Here's the drawing with two shaded views (mm, measured from the low corner). I have some questions. Give positions to 0.01 mm unless a question says otherwise; leave off trailing zeros. Loops run counter-clockwise (first coordinate to the right, second up) from the corner with the lowest first, then second, coordinate; pieces in that order, holes last. Notation, with made-up numbers: (-26.75, 48.5) - (-5.75, 48.5) arc R9 cw to (-5.75, 54.5) - close; hole circle Ø11 at (-27.5, 72.25). An arc over 180 degrees is marked (long way). Write each question's results on one line, items separated by ' | '. Start each with the question number.
1) I want a section at B-B, the plane y = 19. Write out the boundary of the cut face in (x, z).
2) I want a section at C-C, the plane z = 0.6. Write out the boundary of the cut face in (x, y), and give its area (3 significant figures).
3) I'm going to push flat-ended pins straight in: pin 1 (0.7 mm diameter, centred on x = 1.5, z = 2, fed in from +Y); pin 2 (0.9 mm diameter, centred on y = 3.5, z = 2, fed in from -X); pin 3 (0.9 mm diameter, centred on y = 4, z = 2, fed in from +X); pin 4 (1.4 mm diameter, centred on x = 39, y = 22.5, fed in from +Z). Where does each tip first touch, or does it pass through?
4) I want a section at D-D, the plane y = 42. Write out the boundary of the cut face in (x, z), and give its area (3 significant figures).
5) I want a section at A-A, the plane x = 12.5. Write out the boundary of the cut face in (y, z), and give its area (3 significant figures).
6) If I drill on probe 1 along Y at (x, z) = (21, 0.9); probe 2 along X at (y, z) = (35.5, 1.6); probe 3 along Y at (x, z) = (25, 0.2), over which ranges is the centre line in solid material (lowest first)? Write a range as [from, to].
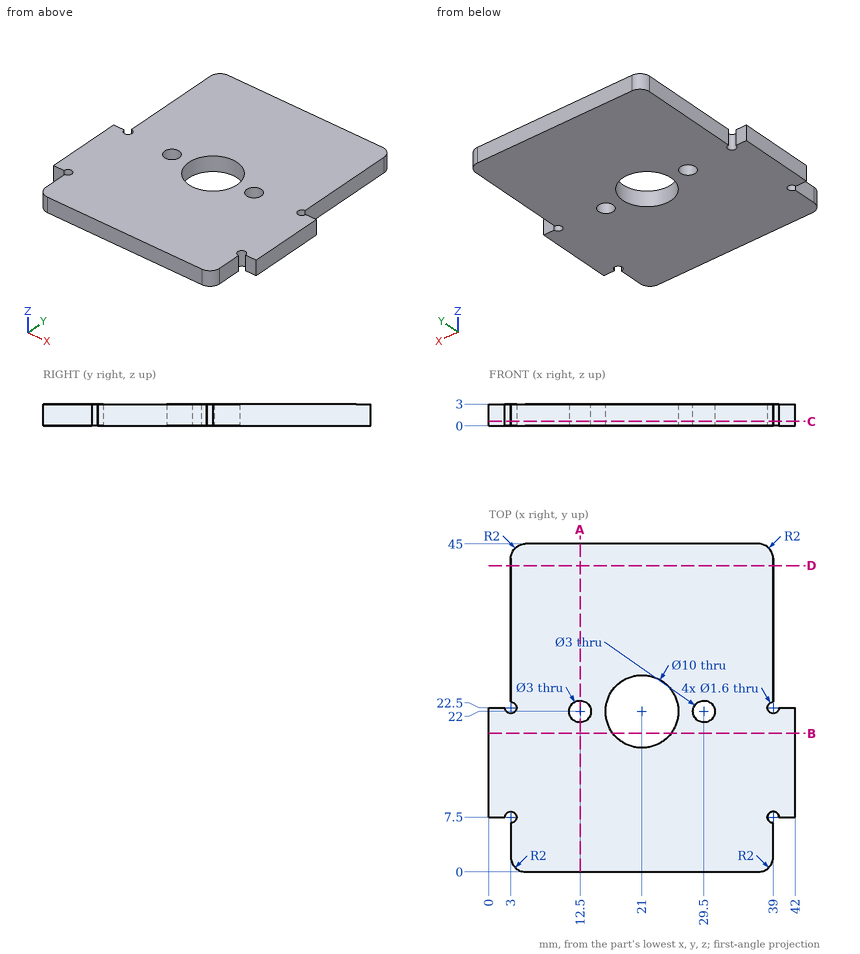
Answers:
1) outline: (0, 0) - (17, 0) - (17, 3) - (0, 3) - close; (25, 0) - (42, 0) - (42, 3) - (25, 3) - close
2) outline: (0, 7.5) - (2.2, 7.5) arc R0.8 cw (long way) to (3, 6.7) - (3, 2) arc R2 ccw to (5, 0) - (37, 0) arc R2 ccw to (39, 2) - (39, 6.7) arc R0.8 cw (long way) to (39.8, 7.5) - (42, 7.5) - (42, 22.5) - (39.8, 22.5) arc R0.8 cw (long way) to (39, 23.3) - (39, 43) arc R2 ccw to (37, 45) - (5, 45) arc R2 ccw to (3, 43) - (3, 23.3) arc R0.8 cw (long way) to (2.2, 22.5) - (0, 22.5) - close; hole circle Ø3 at (12.5, 22); hole circle Ø10 at (21, 22); hole circle Ø3 at (29.5, 22) | area: 1,610 mm2
3) pin 1: stops at y = 22.5 | pin 2: stops at x = 3 | pin 3: stops at x = 39 | pin 4: passes through
4) outline: (3, 0) - (39, 0) - (39, 3) - (3, 3) - close | area: 108 mm2
5) outline: (0, 0) - (20.5, 0) - (20.5, 3) - (0, 3) - close; (23.5, 0) - (45, 0) - (45, 3) - (23.5, 3) - close | area: 126 mm2
6) probe 1: y = [0, 17], [27, 45] | probe 2: x = [3, 39] | probe 3: y = [0, 19], [25, 45]
